```python
from build123d import *

# Parameters (mm, degrees)
SKETCH2_R            = 12.7
BOSS_EXTRUDE1_DEPTH  = 25.4
SKETCH3_R            = 15.875
BOSS_EXTRUDE2_DEPTH  = 25.4
SKETCH4_R            = 19.05
BOSS_EXTRUDE3_DEPTH  = 3.175
SKETCH5_R            = 15.875
BOSS_EXTRUDE4_DEPTH  = 3.175
SKETCH6_R            = 19.05
BOSS_EXTRUDE5_DEPTH  = 43.5356
SKETCH7_R            = 25.4
BOSS_EXTRUDE6_DEPTH  = 25.4
SKETCH8_R            = 19.05
BOSS_EXTRUDE7_DEPTH  = 6.35
SKETCH9_R            = 12.7
BOSS_EXTRUDE8_DEPTH  = 25.4
CUT_EXTRUDE1_DEPTH   = 3.175
SKETCH11_R           = 9.525
BOSS_EXTRUDE9_DEPTH  = 3.175
SKETCH12_R           = 12.7
BOSS_EXTRUDE10_DEPTH = 101.6
SKETCH13_R           = 9.525
BOSS_EXTRUDE11_DEPTH = 3.175
SKETCH14_R           = 12.7
BOSS_EXTRUDE12_DEPTH = 3.175


with BuildPart() as part:
    # Sketch2 → Boss-Extrude1 (new body)
    with BuildSketch(Plane.XY):
        Circle(SKETCH2_R)
    extrude(amount=BOSS_EXTRUDE1_DEPTH)

    # Sketch3 → Boss-Extrude2 (add)
    with BuildSketch(Plane.XY.offset(25.4)):
        Circle(SKETCH3_R)
    extrude(amount=BOSS_EXTRUDE2_DEPTH)

    # Sketch4 → Boss-Extrude3 (add)
    with BuildSketch(Plane.XY.offset(50.8)):
        Circle(SKETCH4_R)
    extrude(amount=BOSS_EXTRUDE3_DEPTH)

    # Sketch5 → Boss-Extrude4 (add)
    with BuildSketch(Plane.XY.offset(53.975)):
        Circle(SKETCH5_R)
    extrude(amount=BOSS_EXTRUDE4_DEPTH)

    # Sketch6 → Boss-Extrude5 (add)
    with BuildSketch(Plane.XY.offset(57.15)):
        Circle(SKETCH6_R)
    extrude(amount=BOSS_EXTRUDE5_DEPTH)

    # Sketch7 → Boss-Extrude6 (add)
    with BuildSketch(Plane.XY.offset(100.6856)):
        Circle(SKETCH7_R)
    extrude(amount=BOSS_EXTRUDE6_DEPTH)

    # Sketch8 → Boss-Extrude7 (add)
    with BuildSketch(Plane.XY.offset(126.0856)):
        Circle(SKETCH8_R)
    extrude(amount=BOSS_EXTRUDE7_DEPTH)

    # Sketch9 → Boss-Extrude8 (add)
    with BuildSketch(Plane.XY.offset(132.4356)):
        Circle(SKETCH9_R)
    extrude(amount=BOSS_EXTRUDE8_DEPTH)

    # Sketch10 → Cut-Extrude1 (cut)
    with BuildSketch(Plane(origin=(0, -19.05, 0), x_dir=(-1, 0, 0), z_dir=(0, -1, 0))):
        with BuildLine():
            Line((3.175, -69.3928), (3.175, -88.4428))
            ThreePointArc((3.175, -88.4428), (0, -91.6178), (-3.175, -88.4428))
            Line((-3.175, -88.4428), (-3.175, -69.3928))
            ThreePointArc((-3.175, -69.3928), (0, -66.2178), (3.175, -69.3928))
        make_face()
    extrude(amount=-CUT_EXTRUDE1_DEPTH, mode=Mode.SUBTRACT)

    # Sketch11 → Boss-Extrude9 (add)
    with BuildSketch(Plane(origin=(0, 0, 0), x_dir=(-1, 0, 0), z_dir=(0, 0, -1))):
        Circle(SKETCH11_R)
    extrude(amount=BOSS_EXTRUDE9_DEPTH)

    # Sketch12 → Boss-Extrude10 (add)
    with BuildSketch(Plane(origin=(0, 0, -3.175), x_dir=(-1, 0, 0), z_dir=(0, 0, -1))):
        Circle(SKETCH12_R)
    extrude(amount=BOSS_EXTRUDE10_DEPTH)

    # Sketch13 → Boss-Extrude11 (add)
    with BuildSketch(Plane.XY.offset(157.8356)):
        Circle(SKETCH13_R)
    extrude(amount=BOSS_EXTRUDE11_DEPTH)

    # Sketch14 → Boss-Extrude12 (add)
    with BuildSketch(Plane.XY.offset(161.0106)):
        Circle(SKETCH14_R)
    extrude(amount=BOSS_EXTRUDE12_DEPTH)


solid = part.part
```
Here's how the part is built. I have some questions about the finished solid (model axes, mm). A direction names the side the tool comes from. Coordinates: 2 decimals unless noted, no trailing zeros. Order: outer loops, then holes, each group sorted by start corner. A loop starts at its lowest first (then second) coordinate and runs counter-clockwise, first axis right, second up. Notation, with made-up numbers: (-24, 42.25) -> (-19, 42.25) arc R14 cw to (-19, 46.25) -> close; hole circle Ø8 at (34, 81.25). An arc over 180 degrees is marked (long way). Return JSON: item names as keys, results as strings.
1) Thinking about a two-plate mould opening in Z: for faces 1 (the cylindrical face through (-2.75, -12.4, 12.52)), 2 (the cylindrical face through (-3.441, -15.497, 55.54)), 3 (the flat face through (-7, 11, 25.4)), which applies, +Z half, -Z half, draft (parallel to the pull), parting line (faces both ways), or undercut?
Conclusion:
{"face 1": "draft", "face 2": "undercut", "face 3": "-Z half"}
2) On a 3-axis mill with a long thin cutter (end or side, diameter ignored), from which of +Z, -Z, +X, -X, +Y, -Y can I reach the whole of each face in a straight line? I mean faces 4 (the cylindrical face through (-15.12, -11.59, 78.61)), 5 (the flat face through (5, 9, 157.836)), 6 (the flat face through (0, -15.875, 79)), 7 (the cylindrical face through (-2.75, -12.4, 162.58)). Say none if no direction works.
Conclusion:
{"face 4": "-Z", "face 5": "none", "face 6": "-Y", "face 7": "+Z"}
3) If we section it at A-A on z = -70: List the corners of the cut face in (x, y) for me, plus the area to 3 significant figures.
Conclusion:
{"outline": "circle Ø25.4 at (0, 0)", "area": "507 mm²"}
4) If I drill on probe 1 along Z at (x, y) = (4.5, -10) (3 decimals); probe 2 along Z at (x, y) = (-16, -2.5) (3 decimals); probe 3 along Z at (x, y) = (13, 18.5), over which ranges is the centre line in solid material (lowest first)?
Conclusion:
{"probe 1": "z = -104.775 to -3.175, 0 to 157.836, 161.011 to 164.186", "probe 2": "z = 50.8 to 53.975, 57.15 to 132.436", "probe 3": "z = 100.69 to 126.09"}
5) I'm going to push flat-ended pins straight in: P1, Ø8, axis at x = -18, y = 18, coming from the -Z side; P2, Ø1.5, axis at y = 12.5, z = 111.5, coming from the +X side; P3, Ø4, axis at y = -12.5, z = 71, coming from the -X side. Where does each tip first touch, or does it pass through?
Conclusion:
{"P1": "stops at z = 100.69", "P2": "stops at x = 22.52", "P3": "stops at x = -15.9"}
